Source: CAD feature listing. Evaluate the final solid. Frame: model axes, mm. Give positions to 0.01 mm unless a question says otherwise; leave off trailing zeros. Loops run counter-clockwise (first coordinate to the right, second up) from the corner with the lowest first, then second, coordinate; pieces in that order, holes last. Notation, with made-up numbers: M -13,-25.75 L 40,-25.75 A27 cw 40,-5.75 Z; hole C 50.25,72.5 d4. An arc over 180 degrees is marked long. Answer in a Markdown table with one row per item.
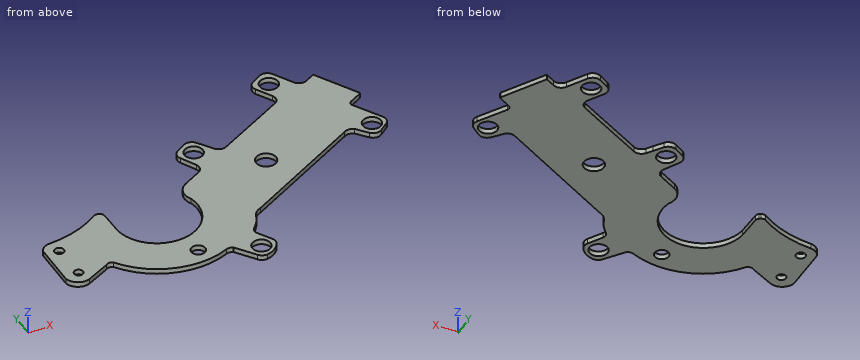
```python
from build123d import *

# Parameters (mm, degrees)
ESBO_O1_R                = 49.227306986
ESBO_O1_R_2              = 45.027223586
ESBO_O1_R_3              = 34.289668097
ESBO_O1_R_4              = 45
ESBO_O1_R_5              = 22.918852427
ESBO_O1_R_6              = 21.929059038
RESSALTO_EXTRUS_O1_DEPTH = 25


with BuildPart() as part:
    # Esboço1 → Ressalto-extrusão1 (new body)
    with BuildSketch(Plane.XY):
        with BuildLine():
            Line((8592.065409332, 5198.475728322), (8473.447242619, 5409.224509958))
            Line((8473.447242619, 5409.224509958), (8425.902270717, 5382.464225227))
            ThreePointArc((8425.902270717, 5382.464225227), (8395.507573393, 5378.800801313), (8371.424844911, 5397.702666012))
            Line((8371.424844911, 5397.702666012), (8316.40665203, 5495.453435889))
            ThreePointArc((8316.40665203, 5495.453435889), (8292.016223819, 5514.440048301), (8261.375488437, 5510.374365776))
            Line((8261.375488437, 5510.374365776), (8212.449282848, 5480.477339997))
            ThreePointArc((8212.449282848, 5480.477339997), (8194.592026382, 5456.406171561), (8198.470371474, 5426.686460968))
            Line((8198.470371474, 5426.686460968), (8241.716603514, 5350.053723792))
            ThreePointArc((8241.716603514, 5350.053723792), (8245.414384596, 5319.663187185), (8226.539756155, 5295.559106588))
            Line((8226.539756155, 5295.559106588), (7887.56689815, 5104.266202112))
            ThreePointArc((7887.56689815, 5104.266202112), (7858.690563236, 5100.178437433), (7834.71418175, 5116.782222212))
            Line((7834.71418175, 5116.782222212), (7814.875485509, 5146.286291727))
            Line((7814.875485509, 5146.286291727), (7784.878848462, 5190.897230564))
            ThreePointArc((7784.878848462, 5190.897230564), (7759.841470177, 5207.737092835), (7730.162808648, 5202.293902357))
            Line((7730.162808648, 5202.293902357), (7684.418563925, 5173.093939339))
            ThreePointArc((7684.418563925, 5173.093939339), (7667.337308495, 5149.854796663), (7670.325681174, 5121.168621105))
            Line((7670.325681174, 5121.168621105), (7709.87388758, 5043.81577039))
            ThreePointArc((7709.87388758, 5043.81577039), (7712.586860583, 5014.16308224), (7694.060285678, 4990.851965593))
            Line((7694.060285678, 4990.851965593), (7603.245211769, 4939.110334103))
            ThreePointArc((7603.245211769, 4939.110334103), (7566.042022636, 4889.986984267), (7574.591315044, 4828.961658539))
            ThreePointArc((7574.591315044, 4828.961658539), (7411.369433565, 4582.346099234), (7179.112865973, 4765.423961074))
            Line((7179.112865973, 4765.423961074), (7179.112865973, 4890.398526732))
            ThreePointArc((7179.112865973, 4890.398526732), (7176.529401806, 4900.23032614), (7169.446438014, 4907.522115401))
            Line((7169.446438014, 4907.522115401), (7161.87645403, 4912.09037363))
            ThreePointArc((7161.87645403, 4912.09037363), (7150.814869868, 4914.953530528), (7139.99090215, 4911.293197972))
            ThreePointArc((7139.99090215, 4911.293197972), (7010.077113446, 4843.731348706), (6866.77493755, 4813.620182095))
            ThreePointArc((6866.77493755, 4813.620182095), (6837.238365249, 4802.28095325), (6817.644330707, 4777.440240208))
            Line((6817.644330707, 4777.440240208), (6812.984670077, 4548.041588809))
            ThreePointArc((6812.984670077, 4548.041588809), (6847.319630156, 4501.148504338), (6905.423739633, 4499.820604987))
            Line((6905.423739633, 4499.820604987), (7018.783227578, 4559.423081996))
            ThreePointArc((7018.783227578, 4559.423081996), (7036.263274842, 4567.468257298), (7054.527862902, 4561.411713646))
            ThreePointArc((7054.527862902, 4561.411713646), (7271.453583291, 4402.062402746), (7539.814575965, 4422.831337767))
            ThreePointArc((7539.814575965, 4422.831337767), (7557.472949269, 4426.146472293), (7574.591376366, 4420.690492236))
            Line((7574.591376366, 4420.690492236), (7643.824786877, 4323.537498877))
            ThreePointArc((7643.824786877, 4323.537498877), (7661.638348099, 4309.574510741), (7684.1782089, 4307.51473498))
            ThreePointArc((7684.1782089, 4307.51473498), (7726.117997258, 4326.065711445), (7756.109950671, 4360.758179011))
            ThreePointArc((7756.109950671, 4360.758179011), (7760.853190032, 4380.173039859), (7755.611379393, 4399.459267136))
            Line((7755.611379393, 4399.459267136), (7714.866132222, 4470.97387784))
            ThreePointArc((7714.866132222, 4470.97387784), (7711.192216927, 4489.765596658), (7719.63329346, 4506.952061587))
            ThreePointArc((7719.63329346, 4506.952061587), (7751.230180611, 4547.174632919), (7772.780877122, 4593.561980354))
            ThreePointArc((7772.780877122, 4593.561980354), (7790.429838997, 4615.627863403), (7814.875485509, 4629.798234485))
            Line((7814.875485509, 4629.798234485), (8402.08207018, 4967.132328945))
            ThreePointArc((8402.08207018, 4967.132328945), (8425.846622391, 4974.638589154), (8449.611174603, 4967.132328945))
            Line((8449.611174603, 4967.132328945), (8495.089773791, 4911.541656895))
            ThreePointArc((8495.089773791, 4911.541656895), (8522.067187452, 4897.068320984), (8551.377293559, 4905.910039154))
            Line((8551.377293559, 4905.910039154), (8593.116417231, 4940.056718911))
            ThreePointArc((8593.116417231, 4940.056718911), (8607.129643298, 4963.786364709), (8602.468925751, 4990.947813611))
            Line((8602.468925751, 4990.947813611), (8523.158682911, 5128.94606196))
            ThreePointArc((8523.158682911, 5128.94606196), (8521.190660044, 5144.12636041), (8530.533149704, 5156.2520547))
            Line((8530.533149704, 5156.2520547), (8594.238523916, 5192.864756379))
            Line((8594.238523916, 5192.864756379), (8592.065409332, 5198.475728322))
        make_face()
        with Locations((7999.136389936, 4936.736467004)):
            Circle(ESBO_O1_R, mode=Mode.SUBTRACT)
        with Locations((8538.305471244, 4970.64052635)):
            Circle(ESBO_O1_R_2, mode=Mode.SUBTRACT)
        with Locations((7428.160556208, 4474.796077944)):
            Circle(ESBO_O1_R_3, mode=Mode.SUBTRACT)
        with Locations((7689.94786831, 4377.665287462)):
            Circle(ESBO_O1_R_4, mode=Mode.SUBTRACT)
        with Locations((6881.727296698, 4746.283471792)):
            Circle(ESBO_O1_R_5, mode=Mode.SUBTRACT)
        with Locations((6883.815097675, 4563.962455068)):
            Circle(ESBO_O1_R_6, mode=Mode.SUBTRACT)
        with Locations((7741.989693859, 5131.410658858)):
            Circle(ESBO_O1_R_4, mode=Mode.SUBTRACT)
        with Locations((8268.711651115, 5436.402584307)):
            Circle(ESBO_O1_R_4, mode=Mode.SUBTRACT)
    extrude(amount=RESSALTO_EXTRUS_O1_DEPTH)


solid = part.part
```
Q1. Section query B-B (x = 6942). Output: boundary loops of the cut face in (y, z), plus the area to 3 significant figures.
Values follow:
| item | result |
|---|---|
| outline | M 4519.05,0 L 4824.33,0 L 4824.33,25 L 4519.05,25 Z |
| area | 7,630 mm^2 |
Q2. Ray query, probe 1 along X at (y, z) = (4547, 10.25); probe 2 along X at (y, z) = (5172, 3); probe 3 along X at (y, z) = (4950, 2.75). Return the intervals inside material, ascending. Write a range as from..to.
Values follow:
| item | result |
|---|---|
| probe 1 | 6813.18..6869.92, 6897.71..6995.16, 7064.48..7751.12 |
| probe 2 | 7682.79..7722.56, 7761.42..7797.59, 8007.59..8557.93 |
| probe 3 | 7622.36..7951.73, 8046.54..8372.26, 8463.63..8498.29, 8578.32..8601.82 |
Q3. Contact query for flat-ended pins moving along their axis: pin 1 Ø5 at (x, y) = (7139, 4746) entering from -Z; pin 2 Ø10 at (x, z) = (8112, 14) entering from +Y; pin 3 Ø2 at (y, z) = (5075, 21.5) entering from +X; pin 4 Ø10 at (x, z) = (8241.5, 11.5) entering from +Y. Output: stop coordinate, or through.
Values follow:
| item | result |
|---|---|
| pin 1 | z = 0 |
| pin 2 | y = 5233.74 |
| pin 3 | x = 8554.74 |
| pin 4 | y = 5501.28 |
Q4. Section query C-C (x = 7245.5). Output: boundary loops of the cut face in (y, z), plus the area to 3 significant figures.
Values follow:
| item | result |
|---|---|
| outline | M 4410.47,0 L 4630.99,0 L 4630.99,25 L 4410.47,25 Z |
| area | 5,510 mm^2 |
Q5. Section query A-A (z = 20.5). Give the number of separate pieces and of enclosed holes in the cut face, plus the area to 3 significant figures.
Values follow:
| item | result |
|---|---|
| separate pieces | 1 |
| enclosed holes | 8 |
| area | 673,000 mm^2 |
